from build123d import *

# Parameters (mm, degrees)
SKETCH1_W           = 20
SKETCH1_H           = 30
BOSS_EXTRUDE1_DEPTH = 15
SKETCH2_R           = 1.8
CUT_EXTRUDE1_DEPTH  = 56.901699437
FILLET2_R           = 5
SKETCH2_3_R         = 2.3
CUT_EXTRUDE2_DEPTH  = 56.901699437
CUT_EXTRUDE3_DEPTH  = 11
SKETCH3_R           = 1.2
CUT_EXTRUDE4_DEPTH  = 11
FILLET3_R           = 10
SKETCH4_R           = 1.5
SKETCH4_W           = 9
SKETCH4_H           = 9
SKETCH4_R_2         = 1.1
CUT_EXTRUDE5_DEPTH  = 3
SKETCH4_2_R         = 1.1
CUT_EXTRUDE6_DEPTH  = 8
SKETCH4_4_R         = 1.5
CUT_EXTRUDE7_DEPTH  = 4
CUT_EXTRUDE8_DEPTH  = 4
SKETCH6_R           = 3.5
SKETCH6_R_2         = 1.8
CUT_EXTRUDE9_DEPTH  = 2.5
CUT_EXTRUDE10_DEPTH = 13.5


with BuildPart() as part:
    # Sketch1 → Boss-Extrude1 (new body)
    with BuildSketch(Plane(origin=(0, 0, 0), x_dir=(1, 0, 0), z_dir=(0, 1, 0))):
        Polygon((-10, 15), (-20, -15), (-10, -15), align=None)
        Rectangle(SKETCH1_W, SKETCH1_H)
        Polygon((10, 15), (20, -15), (10, -15), align=None)
        Polygon((-20, -50), (20, -50), (20, -15), (10, -15), (-10, -15), (-20, -15), align=None)
    extrude(amount=BOSS_EXTRUDE1_DEPTH)

    # Sketch2 → Cut-Extrude1 (cut, through all)
    with BuildSketch(Plane(origin=(0, 15, 0), x_dir=(1, 0, 0), z_dir=(0, 1, 0))):
        with Locations(Location((-12, -9.11, 0), (0, 0, 270))):
            Circle(SKETCH2_R)
        with Locations(Location((12, -9.11, 0), (0, 0, 270))):
            Circle(SKETCH2_R)
        with Locations(Location((-4, 12, 0), (0, 0, 270))):
            Circle(SKETCH2_R)
        with Locations(Location((4, 12, 0), (0, 0, 90))):
            Circle(SKETCH2_R)
    extrude(amount=-CUT_EXTRUDE1_DEPTH, mode=Mode.SUBTRACT)

    # Fillet2
    fillet2_edges = [part.edges().sort_by_distance(p)[0] for p in [
        (-10, 7.5, -15),
        (10, 7.5, -15),
    ]]
    fillet(fillet2_edges, radius=FILLET2_R)

    # Sketch2_3 → Cut-Extrude2 (cut, through all)
    # profile 1 of 2: a face of its own
    with BuildSketch(Plane(origin=(0, 15, 0), x_dir=(1, 0, 0), z_dir=(0, 1, 0))):
        Polygon((-10.666887738, -36.852464686), (-7.72642308, -14.142033875), (4.769272475, -15.75993146), (1.828807817, -38.470362271), align=None)
        with Locations((-3.437427708, -31.637590989)):
            Circle(SKETCH2_3_R, mode=Mode.SUBTRACT)
    # profile 2 of 2: a face of its own
    with BuildSketch(Plane(origin=(0, 15, 0), x_dir=(1, 0, 0), z_dir=(0, 1, 0))):
        with Locations((-3.437427708, -31.637590989)):
            Circle(SKETCH2_3_R)
    extrude(amount=-CUT_EXTRUDE2_DEPTH, mode=Mode.SUBTRACT)

    # Sketch2_4 → Cut-Extrude3 (cut)
    with BuildSketch(Plane(origin=(0, 15, 0), x_dir=(1, 0, 0), z_dir=(0, 1, 0))):
        Polygon((-7.72642308, -14.142033875), (4.769272475, -15.75993146), (5.481917839, -10.255875085), (-7.013777716, -8.6379775), align=None)
        Polygon((1.116162452, -43.974418646), (1.828807817, -38.470362271), (-10.666887738, -36.852464686), (-11.379533103, -42.356521061), align=None)
    extrude(amount=-CUT_EXTRUDE3_DEPTH, mode=Mode.SUBTRACT)

    # Sketch3 → Cut-Extrude4 (cut)
    with BuildSketch(Plane(origin=(0, 4, 0), x_dir=(1, 0, 0), z_dir=(0, 1, 0))):
        with Locations(Location((-1.293710172, -12.504467624, 0), (0, 0, 270))):
            Circle(SKETCH3_R)
        with Locations(Location((-4.863357224, -40.074335595, 0), (0, 0, 270))):
            Circle(SKETCH3_R)
    extrude(amount=-CUT_EXTRUDE4_DEPTH, mode=Mode.SUBTRACT)

    # Fillet3
    fillet3_edges = [part.edges().sort_by_distance(p)[0] for p in [
        (20, 7.5, 50),
        (-20, 7.5, 50),
    ]]
    fillet(fillet3_edges, radius=FILLET3_R)

    # Sketch4 → Cut-Extrude5 (cut)
    # profile 1 of 4: a face of its own
    with BuildSketch(Plane.XY.offset(50)):
        with BuildLine():
            Line((2.90110314, 2.663134509), (10, 2.663134509))
            Line((10, 2.663134509), (10, 11.663134509))
            Line((10, 11.663134509), (2.90110314, 11.663134509))
            add(Edge.make_bspline(
                [(2.90110314, 11.663134509), (2.706802795, 13.50022371), (2.368423756, 15)],
                knots=[5.097231356, 5.097231356, 5.097231356, 5.477961769, 5.477961769, 5.477961769], degree=2, weights=[1, 0.899743473, 0.831672604]))
            Line((2.368423756, 15), (-2.368423756, 15))
            add(Edge.make_bspline(
                [(-2.368423756, 15), (-2.706802795, 13.50022371), (-2.90110314, 11.663134509)],
                knots=[7.088408845, 7.088408845, 7.088408845, 7.469139258, 7.469139258, 7.469139258], degree=2, weights=[0.831672604, 0.899743473, 1]))
            Line((-2.90110314, 11.663134509), (-10, 11.663134509))
            Line((-10, 11.663134509), (-10, 2.663134509))
            Line((-10, 2.663134509), (-2.90110314, 2.663134509))
            add(Edge.make_bspline(
                [(-2.90110314, 2.663134509), (-2.750081515, 1.235241026), (-2.509684133, 0)],
                knots=[1.955638703, 1.955638703, 1.955638703, 2.258324061, 2.258324061, 2.258324061], degree=2, weights=[1, 0.920294828, 0.860932427]))
            Line((-2.509684133, 0), (2.509684133, 0))
            add(Edge.make_bspline(
                [(2.509684133, 0), (2.750081515, 1.235241026), (2.90110314, 2.663134509)],
                knots=[4.024861246, 4.024861246, 4.024861246, 4.327546605, 4.327546605, 4.327546605], degree=2, weights=[0.860932427, 0.920294828, 1]))
        make_face()
        with Locations((0, 7.163134509)):
            Circle(SKETCH4_R, mode=Mode.SUBTRACT)
    # profile 2 of 4: a face of its own
    with BuildSketch(Plane.XY.offset(50)):
        with Locations((0, 7.163134509)):
            Circle(SKETCH4_R)
    # profile 3 of 4: a face of its own
    with BuildSketch(Plane.XY.offset(50)):
        with Locations((14.5, 7.163134509)):
            Rectangle(SKETCH4_W, SKETCH4_H)
        with Locations((14.85, 7.163134509)):
            Circle(SKETCH4_R_2, mode=Mode.SUBTRACT)
    # profile 4 of 4: a face of its own
    with BuildSketch(Plane.XY.offset(50)):
        with Locations((-14.5, 7.163134509)):
            Rectangle(SKETCH4_W, SKETCH4_H)
        with Locations((-14.45, 7.163134509)):
            Circle(SKETCH4_R_2, mode=Mode.SUBTRACT)
    extrude(amount=-CUT_EXTRUDE5_DEPTH, mode=Mode.SUBTRACT)

    # Sketch4_2 → Cut-Extrude6 (cut)
    with BuildSketch(Plane.XY.offset(50)):
        with Locations((-14.45, 7.163134509)):
            Circle(SKETCH4_2_R)
        with Locations((14.85, 7.163134509)):
            Circle(SKETCH4_2_R)
    extrude(amount=-CUT_EXTRUDE6_DEPTH, mode=Mode.SUBTRACT)

    # Sketch4_4 → Cut-Extrude7 (cut)
    with BuildSketch(Plane.XY.offset(50)):
        with Locations((0, 7.163134509)):
            Circle(SKETCH4_4_R)
    extrude(amount=-CUT_EXTRUDE7_DEPTH, mode=Mode.SUBTRACT)

    # Sketch5 → Cut-Extrude8 (cut)
    with BuildSketch(Plane(origin=(0, 4, 0), x_dir=(1, 0, 0), z_dir=(0, 1, 0))):
        with BuildLine():
            Line((-2.435596222, -37.918222619), (-6.402483699, -37.404604338))
            Line((-6.402483699, -37.404604338), (-6.65929284, -39.388048077))
            Line((-6.65929284, -39.388048077), (-5.908796102, -39.485219687))
            ThreePointArc((-5.908796102, -39.485219687), (-4.70927174, -38.884269352), (-3.702354234, -39.770901821))
            Line((-3.702354234, -39.770901821), (-2.692405362, -39.901666358))
            Line((-2.692405362, -39.901666358), (-2.435596222, -37.918222619))
        make_face()
    extrude(amount=-CUT_EXTRUDE8_DEPTH, mode=Mode.SUBTRACT)

    # Sketch6 → Cut-Extrude9 (cut)
    with BuildSketch(Plane.XY.offset(47)):
        with Locations((-5.628460917, 8.8)):
            Circle(SKETCH6_R)
        with Locations((-5.628460917, 8.8)):
            Circle(SKETCH6_R_2, mode=Mode.SUBTRACT)
    extrude(amount=-CUT_EXTRUDE9_DEPTH, mode=Mode.SUBTRACT)

    # Sketch6_2 → Cut-Extrude10 (cut)
    with BuildSketch(Plane.XY.offset(47)):
        with BuildLine():
            ThreePointArc((-3.828460917, 8.8), (-4.355668711, 10.072792206), (-5.628460917, 10.6))
            Line((-5.628460917, 10.6), (-5.628460917, 7))
            ThreePointArc((-5.628460917, 7), (-4.355668711, 7.527207794), (-3.828460917, 8.8))
        make_face()
        with BuildLine():
            Line((-5.628460917, 7), (-5.628460917, 10.6))
            ThreePointArc((-5.628460917, 10.6), (-7.428460917, 8.8), (-5.628460917, 7))
        make_face()
    extrude(amount=-CUT_EXTRUDE10_DEPTH, mode=Mode.SUBTRACT)


solid = part.part
Could you check a few things on this model? Use its own coordinates, in mm. A direction names the side the tool comes from. Give positions to 0.01 mm unless a question says otherwise; leave off trailing zeros. Order: outer loops, then holes, each group sorted by start corner. A loop starts at its lowest first (then second) coordinate and runs counter-clockwise, first axis right, second up. Notation, with made-up numbers: (-35.5, 57) - (17.5, 57) arc R27 cw to (17.5, 83) - close; hole circle Ø8 at (-7.75, 53.5). An arc over 180 degrees is marked (long way). Return JSON: item names as keys, results as strings. Group by question number.
Q1. Suppose I cut it at D-D, the plane z = 0.5. Please give me the cut outline in (x, y), and give its area (3 significant figures).
Q2. Will these pins go through, and if not, where does the flat tip stop? pin 1 Ø0.7 at (x, y) = (-14.5, 6.5) entering from +Z; pin 2 Ø1.5 at (x, z) = (1, 23.5) entering from -Y; pin 3 Ø3.5 at (x, y) = (-6.5, 9) entering from +Z.
Q3. Suppose I cut it at C-C, the plane x = -14.45. Please give me the cut outline in (y, z).
Q4. Thinking about a two-plate mould opening in Z: for faces 1 (the face through (18, 8, 46)), 2 (the face through (-8.505, 2.028, 37.132)), 3 (the face through (-20, 7, 27)), which applies, pulls with the +Z half, pulls with the -Z half, needs draft (parallel to the pull), parting line crosses it, or undercut?
Q5. Which directions (+Z, -Z, +X, -X, +Y, -Y) give clear straight access to the entire face, cutting with the end or side of a thin tool? Please do faces 4 (the face through (-6, 1, 50)), 5 (the face through (-0.2, 8.65, 46.51)), 6 (the face through (-6.53, 2.03, 38.38)), 7 (the face through (-5, 4, 42)).
Q6. Suppose I cut it at A-A, the plane x = 4. Please give me the cut outline in (y, z), and give its area (3 significant figures).
Q7. Suppose I cut it at B-B, the plane x = -5. Please give me the cut outline in (y, z).
Q8. Please list where these lines run through material, in increasing order: line 1 along Y through (x, z) = (-14.45, 43.65); line 2 along X through (y, z) = (8.5, -12); line 3 along X through (y, z) = (2, 35.5). Write a range as [from, to].
Resolved:
{
 "1": {"outline": "(-15.17, 0) - (15.17, 0) - (15.17, 15) - (-15.17, 15) - close", "area": "455 mm2"},
 "2": {"pin 1": "stops at z = 42", "pin 2": "passes through", "pin 3": "stops at z = 44.5"},
 "3": {"outline": "(0, -1.65) - (15, -1.65) - (15, 48.96) - (11.66, 48.96) - (11.66, 47) - (8.26, 47) - (8.26, 42) - (6.06, 42) - (6.06, 47) - (2.66, 47) - (2.66, 48.96) - (0, 48.96) - close"},
 "4": {"face 1": "pulls with the +Z half", "face 2": "undercut", "face 3": "needs draft"},
 "5": {"face 4": "+Z, +X, -X, +Y, -Y", "face 5": "+Z", "face 6": "+Y, -Y", "face 7": "+Y"},
 "6": {"outline": "(0, -15) - (15, -15) - (15, -13.8) - (0, -13.8) - close; (0, -10.2) - (15, -10.2) - (15, 10.06) - (4, 10.06) - (4, 15.66) - (0, 15.66) - close; (0, 21.7) - (15, 21.7) - (15, 50) - (11.66, 50) - (11.66, 47) - (2.66, 47) - (2.66, 50) - (0, 50) - close", "area": "742 mm2"},
 "7": {"outline": "(0, -15) - (15, -15) - (15, -13.5) - (0, -13.5) - close; (0, -10.5) - (15, -10.5) - (15, 8.9) - (4, 8.9) - (4, 14.5) - (0, 14.5) - close; (0, 41.27) - (4, 41.27) - (4, 43.18) - (7.11, 43.18) - (7.11, 44.5) - (5.36, 44.5) - (5.36, 47) - (2.66, 47) - (2.66, 50) - (0, 50) - close; (10.49, 43.18) - (15, 43.18) - (15, 50) - (11.66, 50) - (11.66, 47) - (12.24, 47) - (12.24, 44.5) - (10.49, 44.5) - close"},
 "8": {"line 1": "y = [0, 6.06], [8.26, 15]", "line 2": "x = [-10.98, -5.8], [-2.2, 2.2], [5.8, 10.98]", "line 3": "x = [-20, -10.49], [2.21, 20]"}
}
